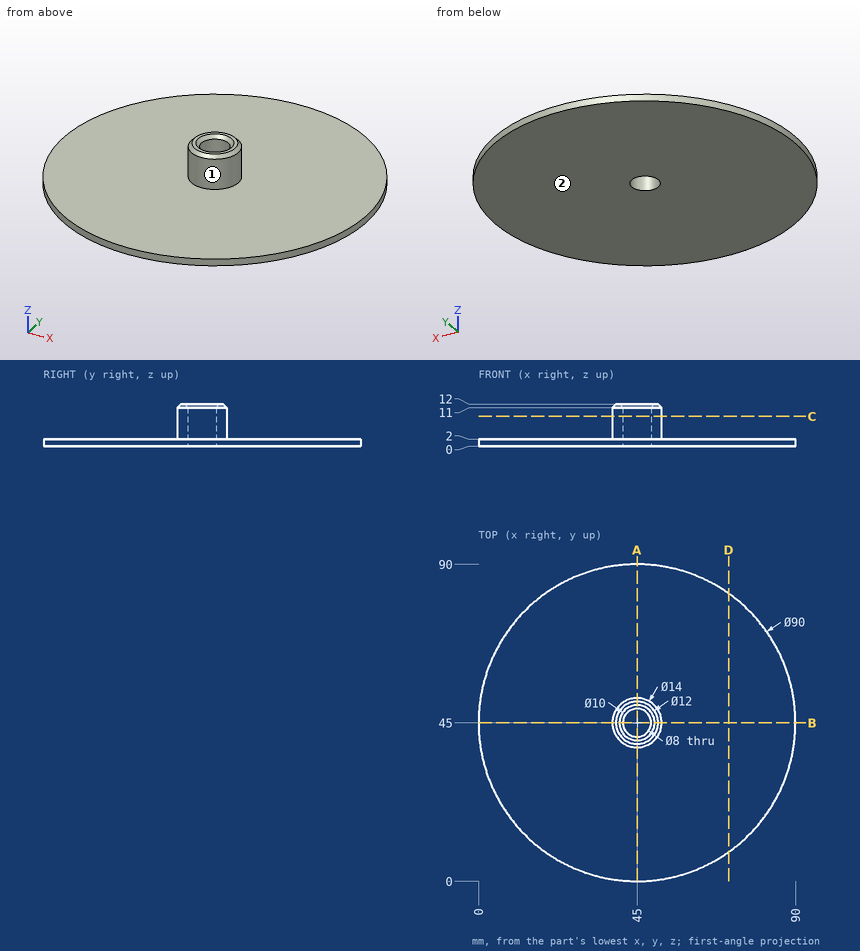
Job drawing, mm, ordinate dimensions from the low corner. One solid piece. A direction names the side the tool comes from. Coordinates: 2 decimals unless noted, no trailing zeros. Order: outer loops, then holes, each group sorted by start corner. A loop starts at its lowest first (then second) coordinate and runs counter-clockwise, first axis right, second up. Notation, with made-up numbers: M 40.25,75.5 L 87.25,75.5 A6 ccw 87.25,81.5 Z; hole C -15,-34 d9. An arc over 180 degrees is marked long. One line per question, with ' | ' between items.
Q1. Pin check, flat tips, straight feed: P1, Ø6, axis at x = 31.5, y = 42.5, coming from the +Z side; P2, Ø5, axis at y = 15.5, z = 2, coming from the -X side. Stop position of each tip, or through.
A:
P1: stops at z = 2 | P2: stops at x = 9
Q2. Slice it at D-D (x = 71). Give the cut face in (y, z).
A:
outline: M 8.27,0 L 81.73,0 L 81.73,2 L 8.27,2 Z
Q3. 3-axis set-ups, long thin cutter, end or side, ignore diameter. For the marked faces 1 and 2: which of +Z, -Z, +X, -X, +Y, -Y reach the whole face in a straight line?
A:
face 1: +Z | face 2: -Z, +X, -X, +Y, -Y
Q4. Slice it at C-C (z = 8.5). Give the cut face in (x, y), and give its area (3 significant figures).
A:
outline: C 45,45 d14; hole C 45,45 d8 | area: 104 mm^2
Q5. Drill centre lines: line 1 (Y direction, x = 45, z = 5.5); line 2 (Z direction, x = 24.5, y = 28). Where is each one in solid material? Low to high.
A:
line 1: y = 38 to 41, 49 to 52 | line 2: z = 0 to 2
Q6. Slice it at A-A (x = 45). Give the cut face in (y, z), and give its area (3 significant figures).
A:
outline: M 0,0 L 41,0 L 41,11 L 40,12 L 39,12 L 38,11 L 38,2 L 0,2 Z; M 49,0 L 90,0 L 90,2 L 52,2 L 52,11 L 51,12 L 50,12 L 49,11 Z | area: 222 mm^2
